For this review, take the finished solid that the model builds, in its own axes (mm). Face numbers are marked on the shaded views. A direction names the side the tool comes from. Round coordinates to 2 decimals unless told otherwise and drop trailing zeros. Order: outer loops, then holes, each group sorted by start corner. A loop starts at its lowest first (then second) coordinate and runs counter-clockwise, first axis right, second up. Notation, with made-up numbers: M 42.5,59 L 68.5,59 A24 cw 68.5,88 Z; hole C -8,84.5 d10. An arc over 180 degrees is marked long. Use a Markdown table: item, result.
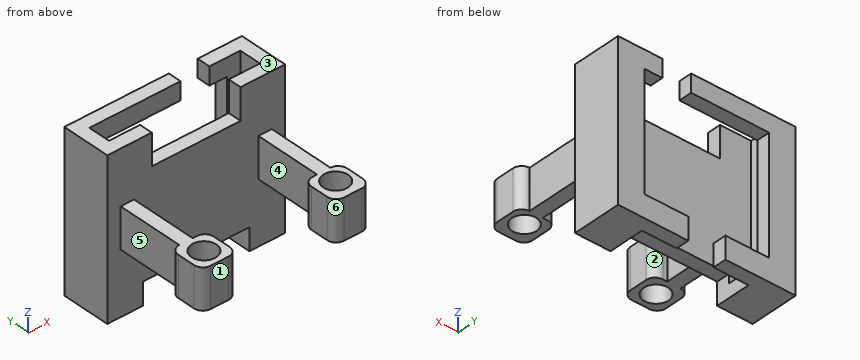
from build123d import *

# Parameters (mm, degrees)
F1_DEPTH  = 1.5
F2_W      = 3
F2_H      = 9
F3_DEPTH  = 15
F4_W      = 2
F4_H      = 9
F5_DEPTH  = 8
F7_D      = 5.6
F8_R      = 1.99999
F9_W      = 5
F9_H      = 3
F10_DEPTH = 3
F12_DEPTH = 2
F13_DEPTH = 2
F14_W     = 3
F14_H     = 4
F14_W_2   = 2
F14_H_2   = 3
F14_W_3   = 9.8253687732
F14_H_3   = 5
F15_DEPTH = 3
F16_W     = 6.5
F16_H     = 4
F17_DEPTH = 3


# Not quite as in the source:
# - a fillet or chamfer is up to 0.001 mm smaller than in the source, because OpenCascade refuses the exact size


with BuildPart() as f1:
    # F0 (on Front) → F1 (new body, symmetric)
    with BuildSketch(Plane.XZ):
        Polygon((-46.7140089311, 21.8801796436), (-46.7140089311, 6.5596503988), (-41.7140089311, 6.5596503988), (-41.7140089311, 8.5596503988), (-29.7140089311, 8.5596503988), (-29.7140089311, 21.8801796436), align=None)
        Polygon((-46.7140089311, 38.5596503988), (-46.7140089311, 21.8801796436), (-29.7140089311, 21.8801796436), (-29.7140089311, 31.5596503988), (-39.7140089311, 31.5596503988), (-39.7140089311, 38.5596503988), align=None)
        Polygon((-12.7140089311, 21.8801796436), (-29.7140089311, 21.8801796436), (-29.7140089311, 8.5596503988), (-17.7140089311, 8.5596503988), (-17.7140089311, 6.5596503988), (-12.7140089311, 6.5596503988), align=None)
        Polygon((-29.7140089311, 31.5596503988), (-29.7140089311, 21.8801796436), (-12.7140089311, 21.8801796436), (-12.7140089311, 38.5596503988), (-19.7140089311, 38.5596503988), (-19.7140089311, 31.5596503988), align=None)
    extrude(amount=F1_DEPTH, both=True)

    # F2 (on face) → F3 (join)
    with BuildSketch(Plane.XZ.offset(1.5)):
        with Locations((-45.2140089311, 22.0596503988)):
            Rectangle(F2_W, F2_H)
        with Locations((-14.2140089311, 22.0596503988)):
            Rectangle(F2_W, F2_H)
    extrude(amount=F3_DEPTH)

    # F4 (on face) → F5 (join)
    with BuildSketch(Plane.XZ.offset(16.5)):
        Polygon((-44.7140089311, 26.5596503988), (-46.7140089311, 26.5596503988), (-46.7140089311, 17.5596503988), (-43.7140089311, 17.5596503988), (-40.7140089311, 17.5596503988), (-40.7140089311, 26.5596503988), (-43.7140089311, 26.5596503988), align=None)
        with Locations((-47.7140089311, 22.0596503988)):
            Rectangle(F4_W, F4_H)
        Polygon((-12.7140089311, 17.5596503988), (-12.7140089311, 26.5596503988), (-14.7140089311, 26.5596503988), (-15.7140089311, 26.5596503988), (-18.7140089311, 26.5596503988), (-18.7140089311, 17.5596503988), (-15.7140089311, 17.5596503988), align=None)
        with Locations((-11.7140089311, 22.0596503988)):
            Rectangle(F4_W, F4_H)
    extrude(amount=F5_DEPTH)

    # F7 (through all)
    with Locations(Plane.XY.offset(26.5596503988)):
        with Locations((-44.7140089311, -20.5), (-14.6104083322, -20)):
            Hole(F7_D / 2)

    # F8 (radius 2 in the source; OpenCascade refuses exactly that, so slightly less here)
    f8_edges = [f1.edges().sort_by_distance(p)[0] for p in [
        (-10.714009, -16.5, 22.05965),
        (-18.714009, -16.5, 22.05965),
        (-18.714009, -24.5, 22.05965),
        (-10.714009, -24.5, 22.05965),
        (-48.714009, -24.5, 22.05965),
        (-48.714009, -16.5, 22.05965),
        (-40.714009, -16.5, 22.05965),
        (-40.714009, -24.5, 22.05965),
    ]]
    fillet(f8_edges, radius=F8_R)

    # F9 (on face) → F10 (join, symmetric)
    with BuildSketch(Plane(origin=(0, 1.5, 0), x_dir=(-1, 0, 0), z_dir=(0, 1, 0))):
        Polygon((12.7140089311, 6.5596503988), (12.7140089311, 38.5596503988), (9.7140089311, 38.5596503988), (9.7140089311, 3.5596503988), (12.7140089311, 3.5596503988), align=None)
        with Locations((15.2140089311, 5.0596503988)):
            Rectangle(F9_W, F9_H)
        with Locations((44.2140089311, 5.0596503988)):
            Rectangle(F9_W, F9_H)
        Polygon((49.7140089311, 38.5596503988), (46.7140089311, 38.5596503988), (46.7140089311, 6.5596503988), (46.7140089311, 3.5596503988), (49.7140089311, 3.5596503988), align=None)
    extrude(amount=F10_DEPTH, both=True)

    # F11 (on face) → F12 (join)
    with BuildSketch(Plane(origin=(0, 4.5, 0), x_dir=(-1, 0, 0), z_dir=(0, 1, 0))):
        Polygon((49.7140089311, 3.5596503988), (49.7140089311, 38.5596503988), (46.7140089311, 38.5596503988), (46.7140089311, 6.5596503988), (41.7140089311, 6.5596503988), (41.7140089311, 3.5596503988), align=None)
    extrude(amount=F12_DEPTH)

    # F13 (add): a face of the model
    f13_faces = [f1.faces().sort_by_distance(p)[0] for p in [
        (-11.7140089311, 4.5, 19.0596503988),
    ]]
    extrude(f13_faces, amount=F13_DEPTH)

    # F14 (on face) → F15 (join)
    with BuildSketch(Plane(origin=(0, 6.5, 0), x_dir=(-1, 0, 0), z_dir=(0, 1, 0))):
        with Locations((48.2140089311, 36.5596503988)):
            Rectangle(F14_W, F14_H)
        Polygon((46.7140089311, 34.5596503988), (46.7140089311, 38.5596503988), (9.7140089311, 38.5596503988), (9.7140089311, 34.5596503988), (15.7140089311, 34.5596503988), (43.7140089311, 34.5596503988), align=None)
        Polygon((49.7140089311, 3.5596503988), (49.7140089311, 34.5596503988), (46.7140089311, 34.5596503988), (46.7140089311, 6.5596503988), (43.7140089311, 6.5596503988), (43.7140089311, 3.5596503988), align=None)
        Polygon((46.7140089311, 6.5596503988), (46.7140089311, 34.5596503988), (43.7140089311, 34.5596503988), (43.7140089311, 8.5596503988), (43.7140089311, 6.5596503988), align=None)
        Polygon((15.7140089311, 34.5596503988), (9.7140089311, 34.5596503988), (9.7140089311, 3.5596503988), (15.7140089311, 3.5596503988), (15.7140089311, 8.5596503988), align=None)
        with Locations((42.7140089311, 5.0596503988)):
            Rectangle(F14_W_2, F14_H_2)
        Polygon((43.7140089311, 6.5596503988), (43.7140089311, 8.5596503988), (33.8886401579, 8.5596503988), (33.8886401579, 3.5596503988), (41.7140089311, 3.5596503988), (41.7140089311, 6.5596503988), align=None)
        with Locations((20.6266933177, 6.0596503988)):
            Rectangle(F14_W_3, F14_H_3)
    extrude(amount=F15_DEPTH)

    # F16 (on face) → F17 (cut)
    with BuildSketch(Plane(origin=(0, 9.5, 0), x_dir=(-1, 0, 0), z_dir=(0, 1, 0))):
        with Locations((22.9359017015, 36.5596503988)):
            Rectangle(F16_W, F16_H)
    extrude(amount=-F17_DEPTH, mode=Mode.SUBTRACT)


solid = f1.part
Q1. Draft analysis for pull direction Y (two halves, no side actions). For the marked faces 1, 2 and 3, state which applies: pulls with the +Y half, pulls with the -Y half, needs draft (parallel to the pull), parting line crosses it, or undercut.
Determined:
| item | result |
|---|---|
| face 1 | pulls with the -Y half |
| face 2 | undercut |
| face 3 | needs draft |
Q2. Add section D-D (x = -30.5). Write out the cut boundary in (y, z), then the cut area to 3 significant figures.
Determined:
| item | result |
|---|---|
| outline | M -1.5,8.56 L 1.5,8.56 L 1.5,31.56 L -1.5,31.56 Z; M 6.5,34.56 L 9.5,34.56 L 9.5,38.56 L 6.5,38.56 Z |
| area | 81.0 mm^2 |
Q3. Machinability: for the marked faces 4, 5 and 6, which of the approach directions +Z, -Z, +X, -X, +Y, -Y give a long, thin tool a straight path to every point of the face, cutting with its end or side? Answer none if there is none.
Determined:
| item | result |
|---|---|
| face 4 | +Z, -Z |
| face 5 | +Z, -Z, -X |
| face 6 | +Z, -Z, -Y |
Q4. Wall thickness on line 1 along X through (y, z) = (8, 36); line 2 along Y through (x, z) = (-45, 35); line 3 along X through (y, z) = (-18, 21): over which ranges is each line inside the solid? List them lowest first. Write a range as [from, to].
Determined:
| item | result |
|---|---|
| line 1 | x = [-49.71, -26.19], [-19.69, -9.71] |
| line 2 | y = [-1.5, 1.5], [6.5, 9.5] |
| line 3 | x = [-48.65, -45.97], [-43.45, -40.78], [-18.65, -16.57], [-12.65, -10.78] |
Q5. Add section B-B (y = -3.5). Write out the cut boundary in (x, z).
Determined:
| item | result |
|---|---|
| outline | M -46.71,17.56 L -43.71,17.56 L -43.71,26.56 L -46.71,26.56 Z; M -15.71,17.56 L -12.71,17.56 L -12.71,26.56 L -15.71,26.56 Z |
Q6. Add section C-C (z = 13). Write out the cut boundary in (x, y), then the cut area to 3 significant figures.
Determined:
| item | result |
|---|---|
| outline | M -49.71,-1.5 L -9.71,-1.5 L -9.71,9.5 L -15.71,9.5 L -15.71,6.5 L -12.71,6.5 L -12.71,1.5 L -46.71,1.5 L -46.71,6.5 L -43.71,6.5 L -43.71,9.5 L -49.71,9.5 Z |
| area | 186 mm^2 |
Q7. Clearance check with flat-ended pins moving along their axes: pin 1 (5 mm diameter, centred on y = -10.5, z = 29, fed in from +X); pin 2 (4 mm diameter, centred on x = -44.5, y = -19.5, fed in from +Z); pin 3 (2.5 mm diameter, centred on x = -15, y = -10.5, fed in from -Z); pin 4 (10 mm diameter, centred on x = -43.5, z = 10.5, fed in from +Y). State where each tip first meets the part, or that it passes through.
Determined:
| item | result |
|---|---|
| pin 1 | stops at x = -12.71 |
| pin 2 | stops at z = 26.56 |
| pin 3 | stops at z = 17.56 |
| pin 4 | stops at y = 9.5 |
Q8. Add section A-A (x = -39). Write out the cut boundary in (y, z).
Determined:
| item | result |
|---|---|
| outline | M -1.5,8.56 L 1.5,8.56 L 1.5,31.56 L -1.5,31.56 Z; M 6.5,3.56 L 9.5,3.56 L 9.5,8.56 L 6.5,8.56 Z; M 6.5,34.56 L 9.5,34.56 L 9.5,38.56 L 6.5,38.56 Z |
